Can you work these out from the drawing? Everything is in mm from the part's minimum corner. A direction names the side the tool comes from. Give positions to 0.01 mm unless a question says otherwise; leave off trailing zeros. Order: outer loops, then holes, each group sorted by start corner. A loop starts at its lowest first (then second) coordinate and runs counter-clockwise, first axis right, second up. Notation, with made-up numbers: (18.5, 37.25) -> (76.5, 37.25) arc R18 cw to (76.5, 62.25) -> close; hole circle Ø11 at (66, 24). An arc over 180 degrees is marked (long way). Answer as CSV lines item,"result". Start each with the question number.
(1) On a 3-axis mill with a long thin cutter (end or side, diameter ignored), from which of +Z, -Z, +X, -X, +Y, -Y can I reach the whole of each face in a straight line? I mean the marked faces 1 and 2. Say none if no direction works.
(2) I need wall thicknesses on L1, parallel to X at y = 12, z = 44; L2, parallel to X at y = 14.75, z = 7.5; L3, parallel to Z at x = 5, y = 14.5. Which ranges of each line are inside material? Lowest first, please.
(3) I want a section at B-B (x = 26). Please give me the cut outline in (y, z).
(4) I want a section at A-A (y = 11.5). Please give me the cut outline in (x, z).
(5) We'd pull the mould along Z, two halves only. Please class the marked faces 3, 4 and 5: released by +Z, released by -Z, zero draft, split by the parting line, or undercut.
(6) Will these pins go through, and if not, where does the flat tip stop? pin 1 Ø1.6 at (x, z) = (12.5, 15) entering from +Y; pin 2 Ø3 at (x, y) = (6.5, 5) entering from -Z; pin 3 Ø5.5 at (y, z) = (18, 57.5) entering from +X.
(7) I want a section at D-D (y = 7.5). Please give me the cut outline in (x, z).
(8) I want a section at C-C (z = 7.5). Please give me the cut outline in (x, y).
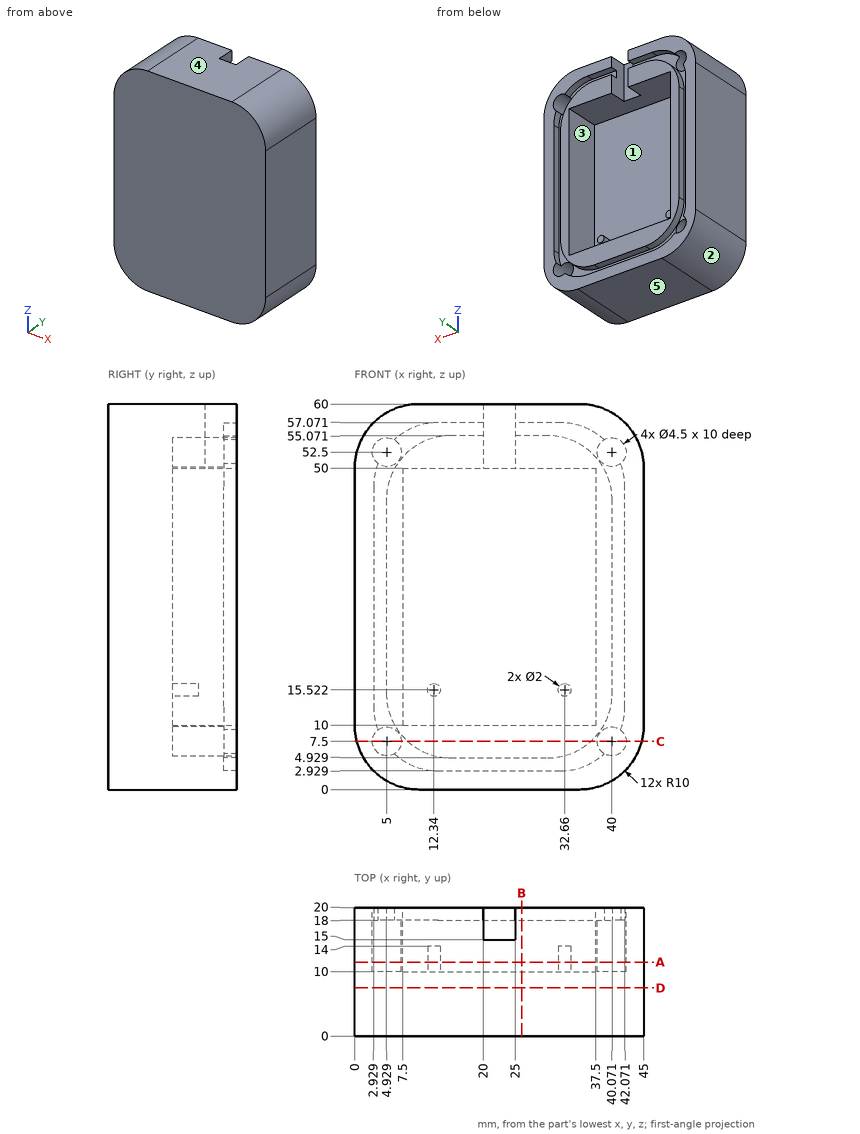
Final values:
1,face 1,"+Y"
1,face 2,"-Z, -X, +Y, -Y"
2,L1,"0 to 7.5, 37.5 to 45"
2,L2,"0.32 to 2.75, 7.25 to 37.75, 42.25 to 44.68"
2,L3,"1.34 to 5.25, 9.75 to 50.25, 54.75 to 58.66"
3,outline,"(0, 0) -> (20, 0) -> (20, 2.93) -> (18, 2.93) -> (18, 4.93) -> (20, 4.93) -> (20, 10) -> (10, 10) -> (10, 50) -> (20, 50) -> (20, 55.07) -> (18, 55.07) -> (18, 57.07) -> (20, 57.07) -> (20, 60) -> (0, 60) -> close"
4,outline,"(0, 10) arc R10 ccw to (10, 0) -> (35, 0) arc R10 ccw to (45, 10) -> (45, 50) arc R10 ccw to (35, 60) -> (10, 60) arc R10 ccw to (0, 50) -> close; circle Ø2 at (12.34, 15.52); circle Ø2 at (32.66, 15.52); hole circle Ø4.5 at (5, 7.5); hole circle Ø4.5 at (5, 52.5); hole (7.5, 10) -> (37.5, 10) -> (37.5, 50) -> (7.5, 50) -> close; hole circle Ø4.5 at (40, 7.5); hole circle Ø4.5 at (40, 52.5)"
5,face 3,"undercut"
5,face 4,"released by +Z"
5,face 5,"released by -Z"
6,pin 1,"y = 14"
6,pin 2,"z = 0.2"
6,pin 3,"x = 43.8"
7,outline,"(0, 10) arc R10 ccw to (10, 0) -> (35, 0) arc R10 ccw to (45, 10) -> (45, 50) arc R10 ccw to (35, 60) -> (10, 60) arc R10 ccw to (0, 50) -> close"
8,outline,"(0.32, 0) -> (44.68, 0) -> (44.68, 20) -> (42.25, 20) -> (42.25, 10) -> (37.75, 10) -> (37.75, 18) -> (36.77, 18) -> (36.77, 20) -> (8.23, 20) -> (8.23, 18) -> (7.25, 18) -> (7.25, 10) -> (2.75, 10) -> (2.75, 20) -> (0.32, 20) -> close"
